Here's how the part is built. I have some questions about the finished solid (model axes, mm). A direction names the side the tool comes from. Round coordinates to 2 decimals unless told otherwise and drop trailing zeros. Loops run counter-clockwise (first coordinate to the right, second up) from the corner with the lowest first, then second, coordinate; pieces in that order, holes last. Notation, with made-up numbers: (48, -13) - (95, -13) arc R27 ccw to (95, 13) - close; hole circle Ø4 at (77.5, -5.5). An arc over 180 degrees is marked (long way). Return JSON: item names as keys, results as strings. Group by question number.
```python
from build123d import *

# Parameters (mm, degrees)
SKETCH1_W           = 190
SKETCH1_H           = 89
BOSS_EXTRUDE1_DEPTH = 4
SKETCH2_W           = 183.6
SKETCH2_H           = 82.6
SKETCH2_W_2         = 179.6
SKETCH2_H_2         = 78.6
BOSS_EXTRUDE2_DEPTH = 4


with BuildPart() as part:
    # Sketch1 → Boss-Extrude1 (new body)
    with BuildSketch(Plane.XY):
        with Locations((-20.5, 3.5)):
            Rectangle(SKETCH1_W, SKETCH1_H)
    extrude(amount=BOSS_EXTRUDE1_DEPTH)

    # Sketch2 → Boss-Extrude2 (add)
    with BuildSketch(Plane(origin=(0, 0, 0), x_dir=(-1, 0, 0), z_dir=(0, 0, -1))):
        with Locations((20.5, 3.5)):
            Rectangle(SKETCH2_W, SKETCH2_H)
        with Locations((20.5, 3.5)):
            Rectangle(SKETCH2_W_2, SKETCH2_H_2, mode=Mode.SUBTRACT)
    extrude(amount=BOSS_EXTRUDE2_DEPTH)


solid = part.part
```
Q1. Imagine slicing it at A-A, the plane z = -1.75. List the corners of the cut face in (x, y) for me, and give its area (3 significant figures).
Q2. Imagine slicing it at B-B, the plane x = -22. List the corners of the cut face in (y, z) for me, and give its area (3 significant figures).
Q3. Imagine slicing it at C-C, the plane y = 14. List the corners of the cut face in (x, z) for me.
Q4. Please list where these lines run through material, in increasing order: line 1 (Y direction, x = -91.5, z = -1.5); line 2 (X direction, y = -6, z = -0.5); line 3 (Z direction, x = 39, y = -19).
Q5. If we mould it in two halves opening along Y, with no side actions, what happens to faces 1 (the flat face through (-20, 43, -4)), 2 (the flat face through (-19, -35.8, -2)), 3 (the flat face through (-19, 44.8, -2))? For each: +Y half, -Y half, draft (parallel to the pull), parting line (faces both ways), or undercut.
Q6. For faces 4 (the flat face through (74.5, 3, 2)), 5 (the flat face through (-112.3, 3, -2)), 6 (the flat face through (-19, -37.8, -2)), 7 (the flat face through (-110.3, 3, -2)), 8 (the flat face through (71.3, 3, -2)), which set-ups out of +Z, -Z, +X, -X, +Y, -Y let a thin tool reach every point of the face, with its end or its side?
Q7. Will these pins go through, and if not, where does the flat tip stop? pin 1 Ø3 at (y, z) = (18.5, -2.5) entering from -X; pin 2 Ø3 at (x, z) = (-44.5, -2) entering from -Y; pin 3 Ø1 at (x, y) = (42, 3) entering from -Z.
Output values:
{
 "1": {"outline": "(-112.3, -37.8) - (71.3, -37.8) - (71.3, 44.8) - (-112.3, 44.8) - close; hole (-110.3, -35.8) - (69.3, -35.8) - (69.3, 42.8) - (-110.3, 42.8) - close", "area": "1,050 mm^2"},
 "2": {"outline": "(-41, 0) - (-37.8, 0) - (-37.8, -4) - (-35.8, -4) - (-35.8, 0) - (42.8, 0) - (42.8, -4) - (44.8, -4) - (44.8, 0) - (48, 0) - (48, 4) - (-41, 4) - close", "area": "372 mm^2"},
 "3": {"outline": "(-115.5, 0) - (-112.3, 0) - (-112.3, -4) - (-110.3, -4) - (-110.3, 0) - (69.3, 0) - (69.3, -4) - (71.3, -4) - (71.3, 0) - (74.5, 0) - (74.5, 4) - (-115.5, 4) - close"},
 "4": {"line 1": "y = -37.8 to -35.8, 42.8 to 44.8", "line 2": "x = -112.3 to -110.3, 69.3 to 71.3", "line 3": "z = 0 to 4"},
 "5": {"face 1": "draft", "face 2": "undercut", "face 3": "+Y half"},
 "6": {"face 4": "+Z, -Z, +X, +Y, -Y", "face 5": "-Z, -X, +Y, -Y", "face 6": "-Z, +X, -X, -Y", "face 7": "-Z", "face 8": "-Z, +X, +Y, -Y"},
 "7": {"pin 1": "stops at x = -112.3", "pin 2": "stops at y = -37.8", "pin 3": "stops at z = 0"}
}
